Source: CAD feature listing. Evaluate the final solid. Frame: model axes, mm. Face numbers are marked on the shaded views. Round coordinates to 2 decimals unless told otherwise and drop trailing zeros. Loops run counter-clockwise (first coordinate to the right, second up) from the corner with the lowest first, then second, coordinate; pieces in that order, holes last. Notation, with made-up numbers: (-23.75, 1) - (30.25, 1) arc R8 ccw to (30.25, 9) - close; hole circle Ø8 at (53.5, 53.5). An arc over 180 degrees is marked (long way). One line per question, with ' | ' between items. Start each with the question number.
1. Cut plane A-A (x = 0). Return loops of the section in (y, z).
2. Pin query (flat end, axial travel): pin 1 (18 mm diameter, centred on x = 8.5, z = 2, fed in from +Y); pin 2 (2 mm diameter, centred on y = 7.5, z = -6, fed in from +X); pin 3 (13.5 mm diameter, centred on x = 0, z = 0, fed in from +Y). Return the tip coordinate at first contact, or that it passes through.
3. Cut plane B-B (z = 0). Return loops of the section in (x, y).
4. Mould query, pull axis Z, two halves, no side actions, for the marked faces 1, 2, 3 and 4. Classes: pulls with the +Z half, pulls with the -Z half, needs draft (parallel to the pull), parting line crosses it, or undercut.
5. Cut plane C-C (y = 6). Return loops of the section in (x, z), then the cut area to 3 significant figures.
6. Ray query, line 1 (Z direction, x = 0, y = 8.95); line 2 (X direction, y = 22.75, z = 0). Return the intervals inside material, ascending.
7. Cut plane D-D (z = 9). Return loops of the section in (x, y), then the cut area to 3 significant figures.
```python
from build123d import *

# Parameters (mm, degrees)
SKETCH2_R               = 24.511
BOSS_EXTRUDE2_DEPTH     = 25.4
SKETCH3_R               = 18.161
CUT_EXTRUDE1_DEPTH      = 12.7
SKETCH11_R              = 83.82
CUT_EXTRUDE2_DEPTH      = 41.402
CUT_EXTRUDE2_DEPTH_BACK = 42.926
SKETCH13_R              = 5.842
CUT_EXTRUDE3_DEPTH      = 42.926
CHAMFER1_SIZE           = 2.032


with BuildPart() as part:
    # Sketch2 → Boss-Extrude2 (new body)
    with BuildSketch(Plane(origin=(0, 0, 0), x_dir=(1, 0, 0), z_dir=(0, 1, 0))):
        Circle(SKETCH2_R)
    extrude(amount=BOSS_EXTRUDE2_DEPTH)

    # Sketch3 → Cut-Extrude1 (cut)
    with BuildSketch(Plane(origin=(0, 25.4, 0), x_dir=(1, 0, 0), z_dir=(0, 1, 0))):
        Circle(SKETCH3_R)
    extrude(amount=-CUT_EXTRUDE1_DEPTH, mode=Mode.SUBTRACT)

    # Sketch11 → Cut-Extrude2 (cut, two sides)
    with BuildSketch(Plane(origin=(0, 0, 0), x_dir=(0, 0, -1), z_dir=(1, 0, 0))) as cut_extrude2_sk:
        with Locations((0, -76.2)):
            Circle(SKETCH11_R)
    extrude(amount=CUT_EXTRUDE2_DEPTH, mode=Mode.SUBTRACT)
    extrude(cut_extrude2_sk.sketch, amount=-CUT_EXTRUDE2_DEPTH_BACK, mode=Mode.SUBTRACT)

    # Sketch13 → Cut-Extrude3 (cut)
    with BuildSketch(Plane(origin=(0, 12.7, 0), x_dir=(1, 0, 0), z_dir=(0, 1, 0))):
        Circle(SKETCH13_R)
    extrude(amount=-CUT_EXTRUDE3_DEPTH, mode=Mode.SUBTRACT)

    # Chamfer1
    chamfer1_edges = [part.edges().sort_by_distance(p)[0] for p in [
        (-5.842, 12.7, 0),
    ]]
    chamfer(chamfer1_edges, length=CHAMFER1_SIZE)


solid = part.part
```
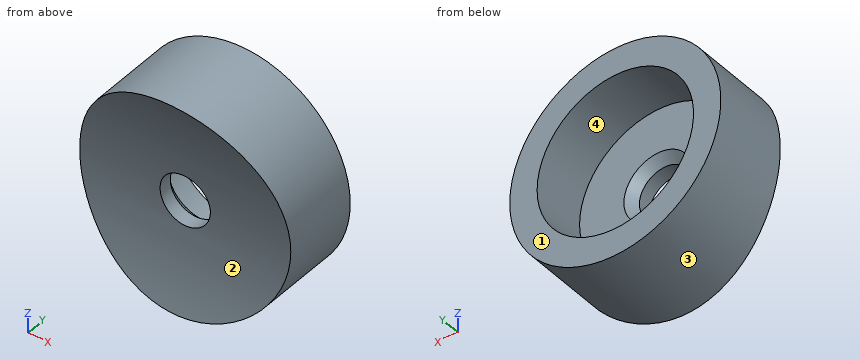
Answers follow:
1) outline: (3.96, -24.51) - (25.4, -24.51) - (25.4, -18.16) - (12.7, -18.16) - (12.7, -7.87) - (10.67, -5.84) - (7.42, -5.84) arc R83.82 cw to start; (3.96, 24.51) arc R83.82 cw to (7.42, 5.84) - (10.67, 5.84) - (12.7, 7.87) - (12.7, 18.16) - (25.4, 18.16) - (25.4, 24.51) - close
2) pin 1: stops at y = 12.7 | pin 2: stops at x = 24 | pin 3: stops at y = 11.58
3) outline: (-24.51, 7.62) - (-5.84, 7.62) - (-5.84, 10.67) - (-7.87, 12.7) - (-18.16, 12.7) - (-18.16, 25.4) - (-24.51, 25.4) - close; (5.84, 7.62) - (24.51, 7.62) - (24.51, 25.4) - (18.16, 25.4) - (18.16, 12.7) - (7.87, 12.7) - (5.84, 10.67) - close
4) face 1: needs draft | face 2: undercut | face 3: parting line crosses it | face 4: undercut
5) outline: (-18.22, -16.4) arc R24.51 ccw to (18.22, -16.4) - close; (-18.22, 16.4) - (18.22, 16.4) arc R24.51 ccw to start | area: 409 mm2
6) line 1: z = -24.51 to -5.84, 5.84 to 24.51 | line 2: x = -24.51 to -18.16, 18.16 to 24.51
7) outline: (-22.8, 7.14) - (22.8, 7.14) - (22.8, 25.4) - (15.77, 25.4) - (15.77, 12.7) - (-15.77, 12.7) - (-15.77, 25.4) - (-22.8, 25.4) - close | area: 432 mm2
